Read the model definition and answer for the solid it produces. Units are mm, in the model's axes. A direction names the side the tool comes from. Give positions to 0.01 mm unless a question says otherwise; leave off trailing zeros. Write each loop counter-clockwise with the first axis right and the second up, starting at its lowest first coordinate (ties: lowest second). Pieces come first, ordered by that corner, then holes. Notation, with made-up numbers: (3, 54) -> (51, 54) arc R16 cw to (51, 80) -> close; hole circle Ø2 at (69.5, -4.5). An arc over 180 degrees is marked (long way). Answer as CSV lines item,"result". Start each with the question number.
1. The part is cut by section D-D, the plane z = 3.5. Determine the outline of the cut face in (x, y), and give its area (3 significant figures).
2. The part is cut by section C-C, the plane y = -20. Determine the outline of the cut face in (x, z), and give its area (3 significant figures).
3. Find the intervals of material crossed by line 1 (Z direction, x = 1.2, y = -20); line 2 (Y direction, x = 20, z = 2.1); line 3 (X direction, y = -13.5, z = 6.75), in increasing order.
4. A tool of negligible diameter and unlimited length cuts with its end or side. For faces 1 (the flat face through (17, -17, 4)), 2 (the flat face through (8, -30, 2.6)), from which of +Z, -Z, +X, -X, +Y, -Y can it reach the whole face along a straight path? Write none if from no direction.
5. Given pin 1 (1 mm diameter, centred on x = 10.5, y = -8, fed in from +Z); pin 2 (4.5 mm diameter, centred on x = 20, z = 23, fed in from +Y); pin 3 (5 mm diameter, centred on x = 20, z = 22.5, fed in from -Y); pin 4 (5 mm diameter, centred on y = -21, z = 11.5, fed in from +X), each flat-ended and moving along its own axis, determine where each tip first touches the part or whether it passes through.
6. The part is cut by section B-B, the plane z = 23. Determine the outline of the cut face in (x, y).
7. For a pull along Y with two mould halves and no side action, classify faces 3 (the flat face through (29.5, -17.2, 3.5)), 4 (the cylindrical face through (2, -22, 9.5)), 5 (the flat face through (0.7, -0.6, 0.7)) as pulls with the +Y half, pulls with the -Y half, needs draft (parallel to the pull), parting line crosses it, or undercut.
8. The part is cut by section A-A, the plane x = 20. Determine the outline of the cut face in (y, z).
from build123d import *

# Parameters (mm, degrees)
SKETCH_W           = 30
SKETCH_H           = 30
PAD_DEPTH          = 30
THICKNESS_T        = -4
SKETCH001_R        = 2.5
POCKET_DEPTH       = 5
POLARPATTERN_COUNT = 2
POLARPATTERN_ANGLE = 90
CYLINDER_R         = 2.5
CYLINDER_DEPTH     = 10
CHAMFER_SIZE       = 8
CHAMFER001_SIZE    = 1


with BuildPart() as part:
    # Sketch → Pad (new body)
    with BuildSketch(Plane.XY):
        with Locations((15, -15)):
            Rectangle(SKETCH_W, SKETCH_H)
    extrude(amount=PAD_DEPTH)

    # Thickness
    thickness_openings = [part.faces().sort_by_distance(p)[0] for p in [
        (30, -15, 15),
        (15, -30, 15),
        (15, -15, 30),
    ]]
    offset(amount=THICKNESS_T, openings=thickness_openings)

    # Sketch001 → Pocket (cut, symmetric)
    with BuildSketch(Plane(origin=(0, 0, 2), x_dir=(0, 1, 0), z_dir=(1, 0, 0))):
        with Locations((-20, 21)):
            Circle(SKETCH001_R)
        with Locations((-20, 9)):
            Circle(SKETCH001_R)
    pocket = extrude(amount=POCKET_DEPTH, both=True, mode=Mode.SUBTRACT)

    # PolarPattern: Pocket ×2 about axis
    polarpattern_axis = Axis((0, 0, 2), (0, 0, 1))
    for i in range(1, POLARPATTERN_COUNT):
        add(pocket.rotate(polarpattern_axis, i * POLARPATTERN_ANGLE / (POLARPATTERN_COUNT - 1)), mode=Mode.SUBTRACT)

    # Cylinder → Cylinder (cut)
    with BuildSketch(Plane(origin=(20, -20, 0), x_dir=(1, 0, 0), z_dir=(0, 0, 1))):
        Circle(CYLINDER_R)
    extrude(amount=CYLINDER_DEPTH, mode=Mode.SUBTRACT)

    # Chamfer
    chamfer_edges = [part.edges().sort_by_distance(p)[0] for p in [
        (4, -4, 17),
    ]]
    chamfer(chamfer_edges, length=CHAMFER_SIZE)

    # Chamfer001
    chamfer001_edges = [part.edges().sort_by_distance(p)[0] for p in [
        (4, -21, 30),
        (8, -8, 30),
        (2, -30, 30),
        (21, -4, 30),
        (30, -2, 30),
        (4, -21, 4),
        (4, -12, 17),
        (4, -30, 17),
        (8, -8, 4),
        (12, -4, 17),
        (30, -30, 2),
        (17, -30, 4),
        (21, -4, 4),
        (30, -4, 17),
        (0, -15, 0),
        (0, 0, 15),
        (30, -17, 4),
        (15, 0, 0),
        (2, -17.5, 23),
        (2, -17.5, 11),
        (17.5, -2, 23),
        (17.5, -2, 11),
        (22.5, -20, 2),
    ]]
    chamfer(chamfer001_edges, length=CHAMFER001_SIZE)


solid = part.part
Results found:
1,outline,"(0, -30) -> (4.5, -30) -> (5, -29.5) -> (29, -29.5) -> (29.5, -29) -> (29.5, -5) -> (30, -4.5) -> (30, 0) -> (1, 0) -> (0, -1) -> close; hole circle Ø5 at (20, -20)"
1,area,"855 mm²"
2,outline,"(0, 1) -> (1, 0) -> (17.5, 0) -> (17.5, 4) -> (5, 4) -> (4, 5) -> (4, 8.5) -> (0, 8.5) -> close; (0, 13.5) -> (4, 13.5) -> (4, 20.5) -> (0, 20.5) -> close; (0, 25.5) -> (4, 25.5) -> (4, 29) -> (3, 30) -> (0, 30) -> close; (22.5, 0) -> (30, 0) -> (30, 3) -> (29, 4) -> (22.5, 4) -> close"
2,area,"163 mm²"
3,line 1,"z = 0 to 8.5, 13.5 to 20.5, 25.5 to 30"
3,line 2,"y = -30 to -22.5, -17.5 to 0"
3,line 3,"x = 0 to 4"
4,face 1,"+Z, +X, -Y"
4,face 2,"+Z, -Z, +X, -X, -Y"
5,pin 1,"stops at z = 4"
5,pin 2,"passes through"
5,pin 3,"stops at y = -4"
5,pin 4,"stops at x = 4"
6,outline,"(0, -30) -> (3, -30) -> (4, -29) -> (4, -22.5) -> (0, -22.5) -> close; (0, -17.5) -> (4, -17.5) -> (4, -13) -> (4.71, -11.29) -> (11.29, -4.71) -> (13, -4) -> (17.5, -4) -> (17.5, 0) -> (1, 0) -> (0, -1) -> close; (22.5, -4) -> (29, -4) -> (30, -3) -> (30, 0) -> (22.5, 0) -> close"
7,face 3,"needs draft"
7,face 4,"undercut"
7,face 5,"pulls with the +Y half"
8,outline,"(-30, 0) -> (-22.5, 0) -> (-22.5, 4) -> (-29, 4) -> (-30, 3) -> close; (-17.5, 0) -> (-1, 0) -> (0, 1) -> (0, 8.5) -> (-4, 8.5) -> (-4, 5) -> (-5, 4) -> (-17.5, 4) -> close; (-4, 13.5) -> (0, 13.5) -> (0, 20.5) -> (-4, 20.5) -> close; (-4, 25.5) -> (0, 25.5) -> (0, 30) -> (-3, 30) -> (-4, 29) -> close"
